Build history of the part. All positions in model axes, mm. Face numbers are marked on the shaded views. A direction names the side the tool comes from. Give positions to 0.01 mm unless a question says otherwise; leave off trailing zeros. Loops run counter-clockwise (first coordinate to the right, second up) from the corner with the lowest first, then second, coordinate; pieces in that order, holes last. Notation, with made-up numbers: (79.25, -0.75) -> (85.25, -0.75) arc R35 cw to (85.25, 37.25) -> close; hole circle Ø11 at (-11, -23.75). An arc over 180 degrees is marked (long way). One line per question, with ' | ' between items. Start each with the question number.
(1) 3-axis set-ups, long thin cutter, end or side, ignore diameter. For the marked faces 1, 2, 3, 4 and 5: which of +Z, -Z, +X, -X, +Y, -Y reach the whole face in a straight line?
(2) Drill centre lines: L1, parallel to Z at x = 1, y = 11.5; L2, parallel to X at y = 9, z = 7; L3, parallel to Y at x = 0.85, z = -9.5. Where is each one in solid material? Low to high. Write a range as from..to.
(3) Mould opens along Y. For the marked faces 6, 7 and 8 say: pulls with the +Y half, pulls with the -Y half, needs draft (parallel to the pull), parting line crosses it, or undercut.
(4) Slice it at C-C, the plane y = 8.25. Write the cut outline in (x, z) (3 decimals).
(5) Slice it at A-A, the plane z = 6.15. Write the cut outline in (x, y).
(6) Flat gauge pins, fed straight in: pin 1 Ø1.2 at (x, y) = (3, 1) entering from -Z; pin 2 Ø0.8 at (x, y) = (6, 1.5) entering from +Z; pin 3 Ø0.5 at (x, z) = (-1.5, 3) entering from -Y; pin 4 Ø6 at (x, y) = (2.5, 12) entering from -Z. Where does each tip first touch, or does it go through?
(7) Slice it at B-B, the plane z = -8.5. Write the cut outline in (x, y), then the cut area to 3 significant figures.
Autodesk Inventor part; units mm, degrees
ref_plane "YZ Plane" through (0, 0, 0) normal (1, 0, 0) x (0, 1, 0)
ref_plane "XZ Plane" through (0, 0, 0) normal (0, 1, 0) x (-1, 0, 0)
ref_plane "XY Plane" through (0, 0, 0) normal (0, 0, 1) x (1, 0, 0)
sketch "スケッチ1" plane through (0, 0, 0) normal (1, 0, 0) x (0, 1, 0)
  circle A0 centre (0, 0) radius 4.575
  circle A1 centre (0, 0) radius 3.575
  line L0 (0, 0) -> (0, 6)
  line L1 (0, 6) -> (0, -6)
  line L2 (0, 0) -> (11.5, 0)
  line L3 (11.5, 0) -> (11.5, 9.5)
  line L4 (11.5, 9.5) -> (11.5, -9.5)
  circle A2 centre (11.5, 9.5) radius 1.65
  circle A3 centre (11.5, -9.5) radius 1.65
  line L5 (0, 0) -> (0, 11.25)
  line L6 (0, 11.25) -> (0, -11.25)
  line L7 (-2.5, -11.25) -> (2.5, -11.25)
  line L8 (2.5, -11.25) -> (2.5, 11.25)
  line L9 (2.5, 11.25) -> (-2.5, 11.25)
  line L10 (-2.5, 11.25) -> (-2.5, -11.25)
  line L11 (-2.5, -11.25) -> (2.5, 11.25) construction
  line L12 (2.5, -11.25) -> (-2.5, 11.25) construction
  circle A4 centre (11.5, 9.5) radius 2.5
  circle A5 centre (11.5, -9.5) radius 2.5
  line L13 (2.5, 11.25) -> (11.2899, 11.9912)
  line L14 (2.5, -11.25) -> (11.2899, -11.9912)
  line L15 (14, 9.5) -> (14, -9.5)
  line L16 (0, -3.575) -> (14, -3.575)
  line L17 (0, 3.575) -> (14, 3.575)
  circle A6 centre (0, 0) radius 6
  line L18 (0, 0) -> (0, 6.15)
  line L19 (0, 6.15) -> (0, -6.15)
  circle A7 centre (0, 6.15) radius 1.25
  circle A8 centre (0, -6.15) radius 1.25
  point P0 (0, 4.575)
  point P1 (0, -4.575)
  point P2 (2.5, 3.575)
  point P3 (2.5, 2.5555)
  point P4 (2.5, -2.5555)
  point P5 (2.5, -3.575)
  point P6 (0, 7.4)
  point P7 (0, 4.9)
  point P8 (0, -4.9)
  point P9 (0, -7.4)
  point P10 (2.5, 5.4544)
  point P11 (2.5, -5.4544)
  point P12 (4.8186, 3.575)
  point P13 (4.8186, -3.575)
  point P14 (2.8548, 3.575)
  point P15 (2.8548, -3.575)
  dimension "d0" = 9.15
  dimension "d1" = 7.15
  dimension "d2" = 6
  dimension "d3" = 12
  dimension "d6" = 11.5
  dimension "d7" = 9.5
  dimension "d8" = 19
  dimension "d9" = 3.3
  dimension "d10" = 3.3
  dimension "d11" = 11.25
  dimension "d12" = 22.5
  dimension "d13" = 5
  dimension "d14" = 5
  dimension "d15" = 5
  dimension "d28" = 12
  dimension "d29" = 6.15
  dimension "d30" = 12.3
  dimension "d31" = 2.5
  dimension "d32" = 2.5
extrude "押し出し7" add sketch "スケッチ1" along normal blind 2 contours L2 A6 L16 A0 | A0 L17 A6 L2 | A0 L8 A6 L17 | L16 A6 L8 A0 | A6 L17 L3 L2 | L2 L4 L16 A6 | A0 L0 A7 A6 L8 | A6 L8 L13 A4 L3 L17 | L8 A6 A8 L1 A0 | L16 L4 A5 L14 L8 A6 | L3 L17 L15 L16 L4 | A6 A7 L5 L9 L8 | L3 A4 L15 L17 | L8 L7 L6 A8 A6 | L16 L15 A5 L4 | A4 | A5
extrude "押し出し8" add sketch "スケッチ1" along normal blind 10 contours L2 A6 L16 A0 | A0 L17 A6 L2 | A0 L8 A6 L17 | L16 A6 L8 A0 | A6 L17 L3 L2 | L2 L4 L16 A6 | A0 L0 A7 A6 L8 | L8 A6 A8 L1 A0 | L3 L17 L15 L16 L4 | A6 A7 L5 L9 L8 | L8 L7 L6 A8 A6
sketch "スケッチ6" plane through (10, 0, 0) normal (1, 0, 0) x (0, 0, -1)
  line L0 (0, 0) -> (-6.15, 0)
  line L1 (-6.15, 0) -> (6.15, 0)
  circle A0 centre (-6.15, 0) radius 1.25
  circle A1 centre (6.15, 0) radius 1.25
  line L2 (-11.25, 2.5) -> (11.25, 2.5)
  line L3 (11.25, 2.5) -> (11.25, -2.5)
  line L4 (11.25, -2.5) -> (-11.25, -2.5)
  line L5 (-11.25, -2.5) -> (-11.25, 2.5)
  line L6 (-11.25, 2.5) -> (11.25, -2.5) construction
  line L7 (11.25, 2.5) -> (-11.25, -2.5) construction
  line L8 (0, 0) -> (0, 11.5)
  line L9 (0, 11.5) -> (-9.5, 11.5)
  line L10 (-9.5, 11.5) -> (9.5, 11.5)
  circle A2 centre (-9.5, 11.5) radius 1.65
  circle A3 centre (-9.5, 11.5) radius 2.5
  circle A4 centre (9.5, 11.5) radius 1.65
  circle A5 centre (9.5, 11.5) radius 2.5
  circle A6 centre (0, 0) radius 6
  circle A7 centre (0, 0) radius 4.575
  arc A8 (11.9912, 11.2899) -> (9.5, 14) centre (9.5, 11.5) ccw
  line L11 (11.25, 2.5) -> (11.9912, 11.2899)
  line L12 (-11.9912, 11.2899) -> (-11.25, 2.5)
  line L13 (-11.25, 2.5) -> (-11.9912, 11.2899)
  line L14 (9.5, 14) -> (-9.5, 14)
  arc A9 (-9.5, 14) -> (-11.9912, 11.2899) centre (-9.5, 11.5) ccw
  line L15 (-9.5, 14) -> (9.5, 14)
  circle A10 centre (0, 0) radius 3.575
  line L16 (-3.575, 14) -> (-3.575, 4.8186)
  line L17 (3.575, -14) -> (-3.575, -14)
  line L18 (-3.575, -14) -> (-3.575, 14)
  line L19 (-3.575, 14) -> (3.575, 14)
  line L20 (3.575, 14) -> (3.575, -14)
  line L21 (3.575, -14) -> (-3.575, 14) construction
  line L22 (-3.575, -14) -> (3.575, 14) construction
  point P0 (-5.4544, 2.5)
  point P1 (5.4544, 2.5)
  point P2 (7, 11.5)
  point P3 (-7, 11.5)
  point P4 (-3.575, 11.5)
  point P5 (-3.575, 4.8186)
  point P6 (-3.575, 2.5)
  point P7 (-2.5555, 2.5)
  point P8 (2.5555, 2.5)
  point P9 (3.575, 2.5)
  point P10 (3.575, 11.5)
  dimension "d69" = 12
  dimension "d56" = 6.15
  dimension "d57" = 12.3
  dimension "d58" = 2.5
  dimension "d59" = 2.5
  dimension "d62" = 11.5
  dimension "d63" = 9.5
  dimension "d64" = 19
  dimension "d65" = 3.3
  dimension "d66" = 5
  dimension "d67" = 3.3
  dimension "d68" = 5
  dimension "d70" = 9.15
  dimension "d79" = 7.15
extrude "押し出し9" add sketch "スケッチ6" against normal blind 2 contours L2 L12 A3 L9 L16 A6 | L16 L9 L8 A6 | A6 L20 L10 A5 L11 L2 | A6 L8 L10 L20 | L16 L14 L20 L10 L9 | L9 A3 L14 L16 | L20 L14 A5 L10 | A3 | A5
extrude "押し出し10" add sketch "スケッチ1" against normal blind 0.5 contours L2 A6 L16 A0 | A0 L17 A6 L2 | A6 L17 L3 L2 | L2 L4 L16 A6 | L3 L17 L15 L16 L4
sketch "スケッチ7" plane through (-0.5, 0, 0) normal (-1, 0, 0) x (0, 0, 1)
  circle A0 centre (0, 0) radius 3.575
  line L0 (-9.5, 14) -> (9.5, 14)
  line L1 (-3.575, 14) -> (3.575, 14)
  circle A1 centre (0, 0) radius 4.575
  line L2 (-11.25, 0) -> (-11.25, 2.5)
  line L3 (11.25, -2.5) -> (-11.25, -2.5)
  line L4 (-11.25, -2.5) -> (-11.25, 2.5)
  line L5 (-11.25, 2.5) -> (11.25, 2.5)
  line L6 (11.25, 2.5) -> (11.25, -2.5)
  line L7 (11.25, -2.5) -> (-11.25, 2.5) construction
  line L8 (-11.25, -2.5) -> (11.25, 2.5) construction
  line L9 (-3.575, 14) -> (-3.575, 0)
  line L10 (3.575, 14) -> (3.575, 0)
  point P0 (-3.575, 2.5)
  point P1 (-2.5555, 2.5)
  point P2 (2.5555, 2.5)
  point P3 (3.575, 2.5)
  dimension "d75" = 7.15
  dimension "d76" = 5
extrude "押し出し11" add sketch "スケッチ7" along normal blind 3 contours A0 L5 L9 A1 L10 | A1 L9 L0 L10
extrude "押し出し12" add sketch "スケッチ6" along normal blind 3 contours L2 L18 A7 L8 A10 | A10 L8 A7 L20 L2 | L18 A6 L8 A7 | A7 L8 A6 L20 | L16 L9 L8 A6 | A6 L8 L10 L20 | L16 L14 L20 L10 L9
properties part number "ikafly3.4c"
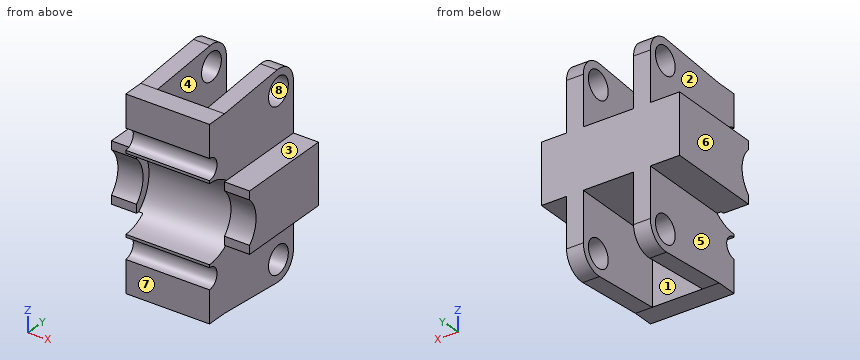
Final values:
1) face 1: -Z, +Y | face 2: +Z, -X, +Y, -Y | face 3: +Z, +X, +Y, -Y | face 4: +Z, +Y | face 5: -Z, -X, +Y, -Y
2) L1: -12..-11.15, -7.85..7.85, 11.15..12 | L2: 0..2, 8..10 | L3: 0..9.85, 13.15..14
3) face 6: needs draft | face 7: pulls with the -Y half | face 8: undercut
4) outline: (-3.5, -3.575) -> (0, -3.575) -> (0, -11.735) -> (2, -11.735) -> (2, -3.575) -> (8, -3.575) -> (8, -11.735) -> (10, -11.735) -> (10, -3.575) -> (13, -3.575) -> (13, 3.575) -> (10, 3.575) -> (10, 11.735) -> (8, 11.735) -> (8, 3.575) -> (2, 3.575) -> (2, 11.735) -> (0, 11.735) -> (0, 3.575) -> (-3.5, 3.575) -> close
5) outline: (0, 1.25) -> (10, 1.25) -> (10, 14) -> (8, 14) -> (8, 2.5) -> (2, 2.5) -> (2, 14) -> (0, 14) -> close
6) pin 1: z = -11.25 | pin 2: z = 11.25 | pin 3: y = 2.5 | pin 4: z = -12
7) outline: (0, 0) -> (10, 0) -> (10, 10.19) -> (8, 10.19) -> (8, 2.5) -> (2, 2.5) -> (2, 10.19) -> (0, 10.19) -> close; (0, 12.81) -> (2, 12.81) -> (2, 14) -> (0, 14) -> close; (8, 12.81) -> (10, 12.81) -> (10, 14) -> (8, 14) -> close | area: 60.5 mm2
